Autodesk Fusion 360 part; units mm, degrees
sketch "Sketch1" plane through (0, 0, 0) normal (0, 0, 1) x (1, 0, 0)
  circle A0 centre (0, 0) radius 14
  circle A1 centre (0, 0) radius 16
  circle A2 centre (0, 0) radius 6.5
  dimension "d1" = 28
  dimension "d2" = 2
  dimension "d10" = 13
extrude "Extrude4" add sketch "Sketch1" along normal blind 10 contours A0
sketch "Sketch2" plane through (0, 0, 10) normal (0, 0, 1) x (-1, 0, 0)
  circle A0 centre (0, 0) radius 14
  circle A1 centre (0, 0) radius 11.1
  circle A2 centre (0, 0) radius 6.5
  circle A3 centre (0, 0) radius 6.5
  circle A4 centre (0, 0) radius 14
  circle A5 centre (0, 0) radius 6.5
  circle A6 centre (0, 0) radius 14
  dimension "d7" = 22.2
extrude "Extrude5" cut sketch "Sketch2" against normal blind 7 contours A1
extrude "Extrude6" add sketch "Sketch1" along normal blind 2 contours A1
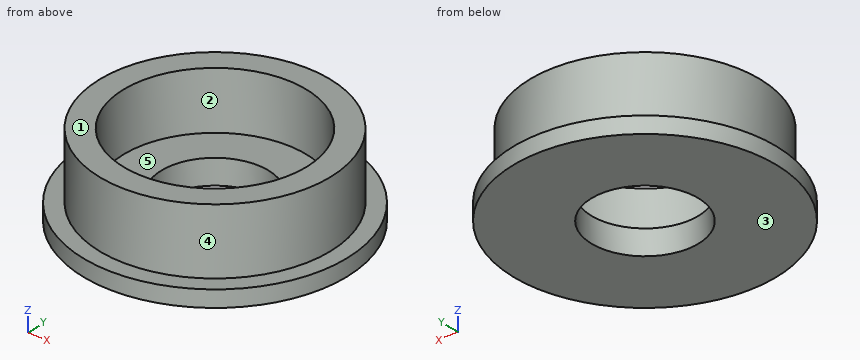
Check sheet for the modelled part. Datum: model origin and axes. Units: mm. Face numbers are marked on the shaded views. A direction names the side the tool comes from. Give positions to 0.01 mm unless a question says otherwise; leave off trailing zeros. Write each loop counter-clockwise with the first axis right and the second up, starting at its lowest first coordinate (ties: lowest second). Pieces come first, ordered by that corner, then holes. Notation, with made-up numbers: (-2.75, 31.5) -> (8.25, 31.5) arc R11 ccw to (8.25, 52.5) -> close; hole circle Ø5 at (69, -37). An arc over 180 degrees is marked (long way). Use CSV: the item, a comma, the result in double quotes. Start each with the question number.
Q1. Cross-section at A-A on x = 0. Enter the section's corners in (y, z), and give its area (3 significant figures).
Q2. Scan lines: line 1 along Y through (x, z) = (0, 7); line 2 along Y through (x, z) = (0, 2.15); line 3 along Z through (x, y) = (14, 7.5). Record each from-to range of solid material in increasing order.
Q3. Cross-section at C-C on z = 4.5. Enter the section's corners in (x, y), and give its area (3 significant figures).
Q4. Release check for a two-part mould opening along Y. For the marked faces 3, 4 and 5 record: +Y half, -Y half, draft (parallel to the pull), parting line (faces both ways), or undercut.
Q5. Depth check by flat-ended pin: P1, Ø1, axis at y = 12, z = 4.5, coming from the -X side; P2, Ø2, axis at x = 10.5, z = 4.5, coming from the +Y side; P3, Ø6, axis at x = 11, z = 6, coming from the -Y side. Enter the tip coordinate at first touch or a pass-through.
Q6. Tool access check on the marked faces 1 and 2. Record the directions out of +Z, -Z, +X, -X, +Y, -Y that give a thin tool (end or side, any length) a straight path to the whole face; none if there is none.
Q7. Cross-section at D-D on x = -12.5. Enter the section's corners in (y, z).
Working result:
1,outline,"(-16, 0) -> (-6.5, 0) -> (-6.5, 3) -> (-11.1, 3) -> (-11.1, 10) -> (-14, 10) -> (-14, 2) -> (-16, 2) -> close; (6.5, 0) -> (16, 0) -> (16, 2) -> (14, 2) -> (14, 10) -> (11.1, 10) -> (11.1, 3) -> (6.5, 3) -> close"
1,area,"93.6 mm^2"
2,line 1,"y = -14 to -11.1, 11.1 to 14"
2,line 2,"y = -14 to -6.5, 6.5 to 14"
2,line 3,"z = 0 to 2"
3,outline,"circle Ø28 at (0, 0); hole circle Ø22.2 at (0, 0)"
3,area,"229 mm^2"
4,face 3,"draft"
4,face 4,"parting line"
4,face 5,"undercut"
5,P1,"stops at x = -7.98"
5,P2,"stops at y = 10.28"
5,P3,"stops at y = -11.49"
6,face 1,"+Z, +X, -X, +Y, -Y"
6,face 2,"+Z"
7,outline,"(-9.99, 0) -> (9.99, 0) -> (9.99, 2) -> (6.3, 2) -> (6.3, 10) -> (-6.3, 10) -> (-6.3, 2) -> (-9.99, 2) -> close"
